```python
from build123d import *

# Parameters (mm, degrees)
BOSS_EXTRUDE1_DEPTH = 9
CUT_EXTRUDE1_DEPTH  = 25
BOSS_EXTRUDE2_DEPTH = 18
LPATTERN1_COUNT     = 5
LPATTERN1_PITCH     = 5
FILLET2_R           = 8
FILLET3_R           = 5
SKETCH7_R           = 1.5
CUT_EXTRUDE2_DEPTH  = 25
SKETCH8_W           = 12
SKETCH8_H           = 17.678618226
CUT_EXTRUDE4_DEPTH  = 8
SKETCH10_R          = 1.75
BOSS_EXTRUDE3_DEPTH = 1.5
SKETCH11_R          = 1.75
BOSS_EXTRUDE5_DEPTH = 1.5
CUT_EXTRUDE5_DEPTH  = 1.5


with BuildPart() as part:
    # Sketch4 → Boss-Extrude1 (new, symmetric)
    with BuildSketch(Plane(origin=(0, 0, 0), x_dir=(0, 0, -1), z_dir=(1, 0, 0))):
        Polygon((110.796991994, 3.426984131), (100.993233908, 1.455607104), (87.193594717, 70.081913709), (110.796991994, 74.426984131), align=None)
        Polygon((126.36598388, -0.864331166), (133.316653042, 6.325119314), (124.689312466, 14.665922308), (112.285585973, 1.836081711), (110.796991994, 3.426984131), (100.993233908, 1.455607104), (96.091354865, 0.469918591), (96.091354865, -9.530081409), (107.980804376, -14.787551363), (115.36598388, -43.864331166), (115.36598388, -50.864331166), (126.36598388, -50.864331166), align=None)
        with BuildLine():
            Line((133.316653042, 6.325119314), (124.689312466, 14.665922308))
            ThreePointArc((124.689312466, 14.665922308), (133.173384251, 14.809191099), (133.316653042, 6.325119314))
        make_face()
    extrude(amount=BOSS_EXTRUDE1_DEPTH, both=True)

    # Sketch5 → Cut-Extrude1 (cut)
    with BuildSketch(Plane(origin=(9, 0, 0), x_dir=(0, 0, -1), z_dir=(1, 0, 0))):
        Polygon((123.66598388, -43.864331166), (123.66598388, -18.864331166), (110.66598388, -18.864331166), align=None)
    extrude(amount=-CUT_EXTRUDE1_DEPTH, mode=Mode.SUBTRACT)

    # Sketch6 → Boss-Extrude2 (add)
    with BuildSketch(Plane(origin=(9, 0, 0), x_dir=(0, 0, -1), z_dir=(1, 0, 0))):
        Polygon((126.36598388, -43.864331166), (130.36598388, -43.864331166), (126.36598388, -41.864331166), align=None)
        Polygon((126.36598388, -43.864331166), (126.36598388, -45.864331166), (130.36598388, -43.864331166), align=None)
    boss_extrude2 = extrude(amount=-BOSS_EXTRUDE2_DEPTH)

    # LPattern1: Boss-Extrude2 ×5
    with Locations(*[(0, i * LPATTERN1_PITCH, 0) for i in range(1, LPATTERN1_COUNT)]):
        add(boss_extrude2)

    # Fillet2
    # the kernel refuses this fillet: 8 mm, written as the material it takes off along each edge
    with BuildSketch(Plane(origin=(-22.024202742, -9.530081409, -96.091354865), x_dir=(0, -0.4044207656516306, -0.9145730393521061), z_dir=(1, 0, 0))) as fillet2_piece_1:
        with BuildLine():
            CenterArc((FILLET2_R * 0.651210137104, FILLET2_R), FILLET2_R, 203.854834431, 66.145165569)
            Line((-FILLET2_R * 0.263362902248, FILLET2_R * 0.595579234348), (-FILLET2_R * 0.281654363035, FILLET2_R * 0.587490819035))
            Line((-FILLET2_R * 0.281654363035, FILLET2_R * 0.587490819035), (-FILLET2_R * 0.0130242027421, -FILLET2_R * 0.02))
            Line((-FILLET2_R * 0.0130242027421, -FILLET2_R * 0.02), (FILLET2_R * 0.651210137104, -FILLET2_R * 0.02))
            Line((FILLET2_R * 0.651210137104, -FILLET2_R * 0.02), (FILLET2_R * 0.651210137104, 0))
        make_face()
    extrude(amount=44.048405484, mode=Mode.SUBTRACT)
    with BuildSketch(Plane(origin=(-24.975146678, 0.469918591, -96.091354865), x_dir=(0, -1, 0), z_dir=(1, 0, 0))) as fillet2_piece_2:
        with BuildLine():
            CenterArc((6.390058671, 8), FILLET2_R, 202.784433835, 67.215566165)
            Line((-0.985688514, 4.901879043), (-1.133203457, 4.839916624))
            ThreePointArc((-1.133203457, 4.839916624), (-0.649704386, 2.419397489), (-0.156860129, -0.031542032))
            Line((-0.156860129, -0.031542032), (0, -0.16))
            Line((0, -0.16), (6.390058671, -0.16))
            Line((6.390058671, -0.16), (6.390058671, 0))
        make_face()
    extrude(amount=49.950293357, mode=Mode.SUBTRACT)

    # Fillet3
    fillet3_edges = [part.edges().sort_by_distance(p)[0] for p in [
        (0, 70.081913709, -87.193594717),
        (0, 74.426984131, -110.796991994),
    ]]
    fillet(fillet3_edges, radius=FILLET3_R)

    # Sketch7 → Cut-Extrude2 (cut)
    with BuildSketch(Plane(origin=(9, 0, 0), x_dir=(0, 0, -1), z_dir=(1, 0, 0))):
        with Locations((93.097450529, 66.084720863)):
            Circle(SKETCH7_R)
    extrude(amount=-CUT_EXTRUDE2_DEPTH, mode=Mode.SUBTRACT)

    # Sketch8 → Cut-Extrude4 (cut)
    with BuildSketch(Plane(origin=(0, 24.86774856, -97.908798117), x_dir=(1, 0, 0), z_dir=(0, -0.246172650114547, 0.9692259934275292))):
        with Locations((0, -57.253709048)):
            Rectangle(SKETCH8_W, SKETCH8_H)
    extrude(amount=-CUT_EXTRUDE4_DEPTH, mode=Mode.SUBTRACT)

    # Sketch10 → Boss-Extrude3 (add)
    with BuildSketch(Plane(origin=(9, 0, 0), x_dir=(0, 0, -1), z_dir=(1, 0, 0))):
        with Locations((129.002982754, 10.495520811)):
            Circle(SKETCH10_R)
    boss_extrude3 = extrude(amount=BOSS_EXTRUDE3_DEPTH)

    # Sketch11 → Boss-Extrude5 (add)
    with BuildSketch(Plane(origin=(9, 0, 0), x_dir=(0, 0, -1), z_dir=(1, 0, 0))):
        with Locations((104.091354865, -4.320400313)):
            Circle(SKETCH11_R)
    boss_extrude5 = extrude(amount=BOSS_EXTRUDE5_DEPTH)

    # Sketch12 → Cut-Extrude5 (cut)
    with BuildSketch(Plane(origin=(9, 0, 0), x_dir=(0, 0, -1), z_dir=(1, 0, 0))):
        with BuildLine():
            Line((105.796991994, 62.137633614), (105.796991994, 19.67893978))
            ThreePointArc((105.796991994, 19.67893978), (105.782233847, 19.507771757), (105.73839501, 19.341655979))
            Line((105.73839501, 19.341655979), (104.874938008, 16.931635031))
            ThreePointArc((104.874938008, 16.931635031), (103.860802938, 16.271567315), (102.953159184, 17.071781129))
            Line((102.953159184, 17.071781129), (94.283666788, 60.185607156))
            ThreePointArc((94.283666788, 60.185607156), (94.435981087, 60.943382118), (95.082997995, 61.366219745))
            Line((95.082997995, 61.366219745), (104.615947394, 63.121108501))
            ThreePointArc((104.615947394, 63.121108501), (105.43689644, 62.906088102), (105.796991994, 62.137633614))
        make_face()
    cut_extrude5 = extrude(amount=-CUT_EXTRUDE5_DEPTH, mode=Mode.SUBTRACT)

    # Mirror1: Boss-Extrude3, Boss-Extrude5, Cut-Extrude5 across plane
    add(boss_extrude3.mirror(Plane(origin=(0, 0, 0), x_dir=(0, 0, 1), z_dir=(1, 0, 0))))
    add(boss_extrude5.mirror(Plane(origin=(0, 0, 0), x_dir=(0, 0, 1), z_dir=(1, 0, 0))))
    add(cut_extrude5.mirror(Plane(origin=(0, 0, 0), x_dir=(0, 0, 1), z_dir=(1, 0, 0))), mode=Mode.SUBTRACT)


solid = part.part
```
The model under review builds one solid part; all positions refer to its coordinate system, in mm. A direction names the side the tool comes from. Coordinates: 2 decimals unless noted, no trailing zeros. Write each loop counter-clockwise with the first axis right and the second up, starting at its lowest first coordinate (ties: lowest second). Pieces come first, ordered by that corner, then holes. Notation, with made-up numbers: (84, -38) -> (110, -38) arc R30 cw to (110, -6) -> close; hole circle Ø2 at (75.5, -30). An arc over 180 degrees is marked (long way). One line per item, written item: value. Start each with the question number.
Q1. Add section B-B, the plane y = 54.5. Give the boundary of the cut face in (x, z), then the cut area to 3 significant figures.
Q2. Add section A-A, the plane z = -119. Give the boundary of the cut face in (x, y), then the cut area to 3 significant figures.
Q3. Clearance check with flat-ended pins moving along their axes: P1, Ø5, axis at x = 4, y = -17, coming from the +Z side; P2, Ø11.5, axis at y = -27.5, z = -116, coming from the +X side; P3, Ø8, axis at x = -4, z = -125, coming from the +Y side. State where each tip first meets the part, or that it passes through.
Q4. To check wall thickness, follow probe 1 along Y at (x, z) = (3.75, -129); probe 2 along Y at (x, z) = (-2.25, -118.5); probe 3 along X at (y, z) = (45, -95.5). State the ranges of each line that lie inside material, in increasing order.
Q5. The part is to be moulded in two halves that separate along Z. For faces 1 (the face through (0.126, -42.878, -128.394)), 2 (the face through (10.5, 11, -129)), 3 (the face through (0.13, 14.9, -133.08)), say which applies: +Z half, -Z half, draft (parallel to the pull), parting line (faces both ways), or undercut.
Q6. For faces 4 (the face through (0, -18.864, -117)), 5 (the face through (9.74, 11.021, -130.672)), 6 (the face through (-9.74, -4.243, -102.343)), 7 (the face through (0.126, -32.878, -128.394)), 8 (the face through (0, -48, -126.366)), list the 3-axis set-ups (+Z, -Z, +X, -X, +Y, -Y) from which the entire face can be reached by the end or side of a thin tool; tool diameter is ignored.
Response:
1. outline: (-9, -110.8) -> (9, -110.8) -> (9, -105.8) -> (7.5, -105.8) -> (7.5, -95.43) -> (9, -95.43) -> (9, -90.33) -> (-9, -90.33) -> (-9, -95.43) -> (-7.5, -95.43) -> (-7.5, -105.8) -> (-9, -105.8) -> close
1. area: 337 mm²
2. outline: (-9, -50.86) -> (9, -50.86) -> (9, -34.89) -> (6, -34.89) -> (6, -37.97) -> (-6, -37.97) -> (-6, -34.89) -> (-9, -34.89) -> close; (-9, -18.86) -> (9, -18.86) -> (9, 8.78) -> (-9, 8.78) -> close
2. area: 748 mm²
3. P1: z = -107.33
3. P2: x = 9
3. P3: y = 16.5
4. probe 1: -44.55 to -43.18, -39.55 to -38.18, -34.55 to -33.18, -29.55 to -28.18, -24.55 to -23.18, 1.86 to 16.5
4. probe 2: -50.86 to -38.09, -18.86 to 8.26
4. probe 3: -9 to 9
5. face 1: -Z half
5. face 2: draft
5. face 3: undercut
6. face 4: +X, -X
6. face 5: +X
6. face 6: -X
6. face 7: -Z, +X, -X
6. face 8: -Z, +X, -X, -Y
